from build123d import *

# Parameters (mm, degrees)
F1_DEPTH = 63.5
F2_DEPTH = 25.4
F3_DEPTH = 3.3655
F0_W     = 25.2081867933
F0_H     = 19.05
F4_DEPTH = 25.4
F6_R     = 5.08


# Not quite as in the source:
# - a feature names something its author has since deleted; it is built from what else it names


with BuildPart() as f1:
    # F0 (on Front) → F1 (new body, symmetric)
    with BuildSketch(Plane.XZ):
        Polygon((-41.275, -9.525), (41.275, -9.525), (41.275, 9.525), (22.225, 9.525), (-41.275, 9.525), align=None)
    extrude(amount=F1_DEPTH, both=True)

    # F0 (on Front) → F2 (join, symmetric)
    with BuildSketch(Plane.XZ):
        with BuildLine():
            Line((22.225, 9.525), (41.275, 9.525))
            Line((41.275, 9.525), (41.275, 26.6985158606))
            ThreePointArc((41.275, 26.6985158606), (46.0130410873, 38.1371589127), (57.4516841394, 42.8752))
            Line((57.4516841394, 42.8752), (60.325, 42.8752))
            Line((60.325, 42.8752), (60.325, 61.9252))
            Line((60.325, 61.9252), (57.4516841394, 61.9252))
            ThreePointArc((57.4516841394, 61.9252), (32.5426569057, 51.6075430943), (22.225, 26.6985158606))
            Line((22.225, 26.6985158606), (22.225, 9.525))
        make_face()
    extrude(amount=F2_DEPTH, both=True)

    # F0 (on Front) → F3 (join, symmetric)
    with BuildSketch(Plane.XZ):
        with BuildLine():
            add(Edge.make_bspline(
                [(-41.275, 9.525), (-40.5068695545, 53.2762855291), (10.412055999, 64.5915940404), (57.4516841394, 61.9252)],
                knots=[0, 0, 0, 0, 111.7709225211, 111.7709225211, 111.7709225211, 111.7709225211], degree=3))
            Line((-41.275, 9.525), (22.225, 9.525))
            Line((22.225, 9.525), (22.225, 26.6985158606))
            ThreePointArc((22.225, 26.6985158606), (32.5426569057, 51.6075430943), (57.4516841394, 61.9252))
        make_face()
    extrude(amount=F3_DEPTH, both=True)

    # F0 (on Front) → F4 (join, symmetric)
    with BuildSketch(Plane.XZ):
        with Locations((72.9290933967, 52.4002)):
            Rectangle(F0_W, F0_H)
    extrude(amount=F4_DEPTH, both=True)

    # F0 (on Front) → F5 (revolve)
    with BuildSketch(Plane.XZ):
        Polygon((85.5331867933, 66.675), (85.5331867933, 61.9252), (85.5331867933, 42.8752), (85.5331867933, 38.1), (111.125, 38.1), (111.125, 66.675), align=None)
    revolve(axis=Axis((85.5331867933, 0, 52.3875), (0, 0, -1)))

    # F6
    f6_edges = [f1.edges().sort_by_distance(p)[0] for p in [
        (41.275, -63.5, 0),
        (-41.275, -63.5, 0),
        (41.275, 63.5, 0),
        (-41.275, 63.5, 0),
    ]]
    fillet(f6_edges, radius=F6_R)


solid = f1.part
Geometry check sheet. Reference: the model listing, model coordinates, mm. A direction names the side the tool comes from. Coordinates: 2 decimals unless noted, no trailing zeros. Loops run counter-clockwise (first coordinate to the right, second up) from the corner with the lowest first, then second, coordinate; pieces in that order, holes last. Notation, with made-up numbers: (9, 64) - (35, 64) arc R22 ccw to (35, 97) - close; hole circle Ø8 at (0, 36). An arc over 180 degrees is marked (long way). Use one line per item in the form item = value. Start each with the question number.
Item 1: Section check A-A, the plane z = 6. Enter the section's corners in (x, y) (3 decimals).
Item 2: Section check B-B, the plane y = -7.5. Enter the section's corners in (x, z) (3 decimals).
Item 3: Tool access check on faces 1 (the face through (22.225, -15, 18)), 2 (the face through (39.8, -62, 0.1)), 3 (the face through (-2, 3.366, 31)), 4 (the face through (85, 0, 66.675)), 5 (the face through (41.275, -1, 4)). Record the directions out of +Z, -Z, +X, -X, +Y, -Y that give a thin tool (end or side, any length) a straight path to the whole face; none if there is none.
Item 4: Section check C-C, the plane y = 41. Enter the section's corners in (x, z) (3 decimals), and give its area (3 significant figures).
Item 5: Mould release check, pull along X, two halves, no side actions. Record for faces 6 (the face through (-39.75, -62.05, -0.13)), 7 (the face through (45, 25.4, 42)), 8 (the face through (59.7, -0.1, 42.875)), 9 (the face through (45.89, -0.36, 38.01)): +X half, -X half, draft (parallel to the pull), parting line (faces both ways), or undercut.
Item 6: Thickness scan on probe 1 along Z at (x, y) = (-34, 5.5) (3 decimals); probe 2 along Y at (x, z) = (3.5, 35); probe 3 along Y at (x, z) = (49, 57.5). Record the ranges inside material, lowest first.
Item 7: Gauge pin test, flat ends, axial feed: pin 1 (6 mm diameter, centred on x = 28, y = -9, fed in from +Z); pin 2 (15.5 mm diameter, centred on x = 51, z = 35, fed in from -Y); pin 3 (15.5 mm diameter, centred on x = 41.5, z = 41, fed in from +Y); pin 4 (3 mm diameter, centred on x = 88, y = -28, fed in from +Z). Record the tip position at first contact, or that the pin passes through.
Computed:
q1.outline = (-41.275, -58.42) arc R5.08 ccw to (-36.195, -63.5) - (36.195, -63.5) arc R5.08 ccw to (41.275, -58.42) - (41.275, 58.42) arc R5.08 ccw to (36.195, 63.5) - (-36.195, 63.5) arc R5.08 ccw to (-41.275, 58.42) - close
q2.outline = (-41.275, -9.525) - (41.275, -9.525) - (41.275, 26.699) arc R16.177 cw to (57.452, 42.875) - (61.065, 42.875) - (61.065, 38.1) - (110.001, 38.1) - (110.001, 66.675) - (61.065, 66.675) - (61.065, 61.925) - (57.452, 61.925) arc R35.227 ccw to (22.225, 26.699) - (22.225, 9.525) - (-41.275, 9.525) - close
q3.face_1 = +Z, -X, -Y
q3.face_2 = +Z, -Z, +X, -Y
q3.face_3 = +Z, -X, +Y
q3.face_4 = +Z, +X, -X, +Y, -Y
q3.face_5 = -Z, +X, +Y, -Y
q4.outline = (-41.275, -9.525) - (41.275, -9.525) - (41.275, 9.525) - (-41.275, 9.525) - close
q4.area = 1,570 mm2
q5.face_6 = -X half
q5.face_7 = draft
q5.face_8 = undercut
q5.face_9 = undercut
q6.probe_1 = -9.525 to 9.525
q6.probe_2 = -3.37 to 3.37
q6.probe_3 = -25.4 to 25.4
q7.pin_1 = 49.96
q7.pin_2 = -25.4
q7.pin_3 = 25.4
q7.pin_4 = through
